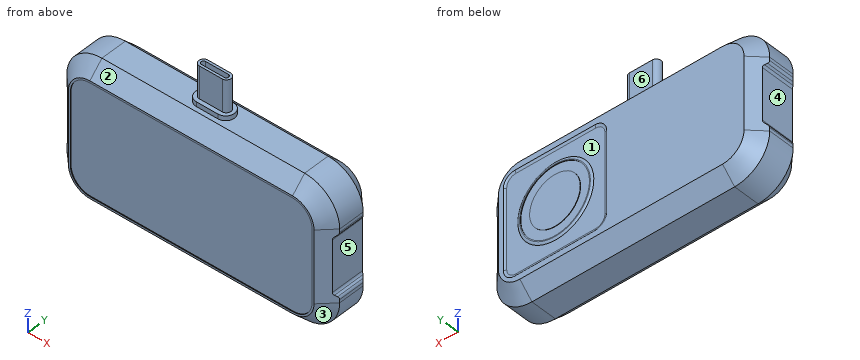
```python
from build123d import *

# Parameters (mm, degrees)
SKETCH1_W               = 70
SKETCH1_H               = 36.5
BOSS_EXTRUDE1_DEPTH     = 6.9
BOSS_EXTRUDE2_DEPTH     = 1.2
BOSS_EXTRUDE3_DEPTH     = 8.25
FILLET1_R               = 9
SKETCH4_R               = 9.75
CUT_EXTRUDE1_DEPTH      = 0.25
SKETCH5_R               = 8.85
SKETCH5_R_2             = 6.5
CUT_EXTRUDE2_DEPTH      = 0.1
CHAMFER1_SIZE           = 3.5
CUT_EXTRUDE3_DEPTH      = 0.2
CUT_EXTRUDE4_DEPTH      = 46.16525213
CUT_EXTRUDE4_DEPTH_BACK = 46.16525213
FILLET2_R               = 1
FILLET3_R               = 1


with BuildPart() as part:
    # Sketch1 → Boss-Extrude1 (new, symmetric)
    with BuildSketch(Plane(origin=(0, 0, 0), x_dir=(1, 0, 0), z_dir=(0, 1, 0))):
        Rectangle(SKETCH1_W, SKETCH1_H)
    extrude(amount=BOSS_EXTRUDE1_DEPTH, both=True)

    # Sketch2 → Boss-Extrude2 (add)
    with BuildSketch(Plane.XY.offset(18.25)):
        with BuildLine():
            Line((2.75, -2.25), (-2.75, -2.25))
            ThreePointArc((-2.75, -2.25), (-5, 0), (-2.75, 2.25))
            Line((-2.75, 2.25), (2.75, 2.25))
            ThreePointArc((2.75, 2.25), (5, 0), (2.75, -2.25))
        make_face()
    extrude(amount=BOSS_EXTRUDE2_DEPTH)

    # Sketch3 → Boss-Extrude3 (add)
    with BuildSketch(Plane.XY.offset(19.45)):
        with BuildLine():
            Line((2.925, -1.2), (-2.925, -1.2))
            ThreePointArc((-2.925, -1.2), (-4.125, 0), (-2.925, 1.2))
            Line((-2.925, 1.2), (2.925, 1.2))
            ThreePointArc((2.925, 1.2), (4.125, 0), (2.925, -1.2))
        make_face()
        with BuildLine():
            Line((2.925, -0.6), (-2.925, -0.6))
            ThreePointArc((-2.925, -0.6), (-3.525, 0), (-2.925, 0.6))
            Line((-2.925, 0.6), (2.925, 0.6))
            ThreePointArc((2.925, 0.6), (3.525, 0), (2.925, -0.6))
        make_face(mode=Mode.SUBTRACT)
    extrude(amount=BOSS_EXTRUDE3_DEPTH)

    # Fillet1
    fillet1_edges = [part.edges().sort_by_distance(p)[0] for p in [
        (35, 0, 18.25),
        (-35, 0, 18.25),
        (-35, 0, -18.25),
        (35, 0, -18.25),
    ]]
    fillet(fillet1_edges, radius=FILLET1_R)

    # Sketch4 → Cut-Extrude1 (cut)
    with BuildSketch(Plane(origin=(0, 6.9, 0), x_dir=(1, 0, 0), z_dir=(0, 1, 0))):
        with BuildLine():
            Line((27.25, 13.25), (6.75, 13.25))
            ThreePointArc((6.75, 13.25), (4.628679656, 12.371320344), (3.75, 10.25))
            Line((3.75, 10.25), (3.75, -10.25))
            ThreePointArc((3.75, -10.25), (4.628679656, -12.371320344), (6.75, -13.25))
            Line((6.75, -13.25), (27.25, -13.25))
            ThreePointArc((27.25, -13.25), (29.371320344, -12.371320344), (30.25, -10.25))
            Line((30.25, -10.25), (30.25, 10.25))
            ThreePointArc((30.25, 10.25), (29.371320344, 12.371320344), (27.25, 13.25))
        make_face()
        with Locations(Location((17, 0, 0), (0, 0, 270))):
            Circle(SKETCH4_R, mode=Mode.SUBTRACT)
    extrude(amount=-CUT_EXTRUDE1_DEPTH, mode=Mode.SUBTRACT)

    # Sketch5 → Cut-Extrude2 (cut)
    with BuildSketch(Plane(origin=(0, 6.9, 0), x_dir=(1, 0, 0), z_dir=(0, 1, 0))):
        with Locations(Location((17, 0, 0), (0, 0, 270))):
            Circle(SKETCH5_R)
        with Locations(Location((17, 0, 0), (0, 0, 270))):
            Circle(SKETCH5_R_2, mode=Mode.SUBTRACT)
    extrude(amount=-CUT_EXTRUDE2_DEPTH, mode=Mode.SUBTRACT)

    # Chamfer1
    chamfer1_edges = [part.edges().sort_by_distance(p)[0] for p in [
        (0, -6.9, -18.25),
        (0, 6.9, -18.25),
        (35, -6.9, 0),
        (0, -6.9, 18.25),
        (-35, -6.9, 0),
        (-32.363961031, -6.9, 15.613961031),
        (-32.363961031, -6.9, -15.613961031),
        (32.363961031, -6.9, 15.613961031),
        (32.363961031, -6.9, -15.613961031),
        (35, 6.9, 0),
        (-35, 6.9, 0),
        (0, 6.9, 18.25),
        (-32.363961031, 6.9, 15.613961031),
        (-32.363961031, 6.9, -15.613961031),
        (32.363961031, 6.9, 15.613961031),
        (32.363961031, 6.9, -15.613961031),
    ]]
    chamfer(chamfer1_edges, length=CHAMFER1_SIZE)

    # Sketch6 → Cut-Extrude3 (cut)
    with BuildSketch(Plane.XZ.offset(6.9)):
        with BuildLine():
            Line((-26, -14.25), (26, -14.25))
            ThreePointArc((26, -14.25), (29.535533906, -12.785533906), (31, -9.25))
            Line((31, -9.25), (31, 9.25))
            ThreePointArc((31, 9.25), (29.535533906, 12.785533906), (26, 14.25))
            Line((26, 14.25), (-26, 14.25))
            ThreePointArc((-26, 14.25), (-29.535533906, 12.785533906), (-31, 9.25))
            Line((-31, 9.25), (-31, -9.25))
            ThreePointArc((-31, -9.25), (-29.535533906, -12.785533906), (-26, -14.25))
        make_face()
    extrude(amount=-CUT_EXTRUDE3_DEPTH, mode=Mode.SUBTRACT)

    # Sketch7 → Cut-Extrude4 (cut, two sides: drawn at the far end of the back side and taken through both)
    with BuildSketch(Plane(origin=(0, 0, 0), x_dir=(1, 0, 0), z_dir=(0, 1, 0)).offset(-CUT_EXTRUDE4_DEPTH_BACK)):
        Polygon((-34, -7), (-34, 7), (-35, 8), (-35, -8), align=None)
        Polygon((34, 7), (35, 8), (35, -8), (34, -7), align=None)
    extrude(amount=CUT_EXTRUDE4_DEPTH + CUT_EXTRUDE4_DEPTH_BACK, mode=Mode.SUBTRACT)

    # Fillet2
    fillet2_edges = [part.edges().sort_by_distance(p)[0] for p in [
        (34, 0, 7),
        (34, 0, -7),
        (35, 0, -8),
        (35, 0, 8),
        (-35, 0, -8),
        (-34, 0, -7),
        (-34, 0, 7),
        (-35, 0, 8),
    ]]
    fillet(fillet2_edges, radius=FILLET2_R)

    # Fillet3
    # the kernel refuses this fillet: 1 mm, written as the material it adds along each edge
    with BuildSketch(Plane(origin=(27.25, 6.65, -10.25), x_dir=(1, 0, 0), z_dir=(0, 0, 1))) as fillet3_piece_1:
        with BuildLine():
            CenterArc((2.338562172, 1), FILLET3_R, 270, 41.409622109)
            Line((2.338562172, 0), (2.338562172, -0.02))
            Line((2.338562172, -0.02), (3, -0.02))
            Line((3, -0.02), (3.02, 0))
            ThreePointArc((3.02, 0), (3.02, 0.125), (3.013228757, 0.235))
            Line((3.013228757, 0.235), (3, 0.25))
        make_face()
    revolve(axis=Axis((27.25, 6.65, -10.25), (0, 1, 0)), revolution_arc=90)
    with BuildSketch(Plane(origin=(30.25, 6.65, 10.25), x_dir=(0, 1, 0), z_dir=(0, 0, -1)), Plane(origin=(6.75, 6.65, 13.25), x_dir=(0, 1, 0), z_dir=(1, 0, 0)), Plane(origin=(3.75, 6.65, -10.25), x_dir=(0, 1, 0), z_dir=(0, 0, 1)), Plane(origin=(27.25, 6.65, -13.25), x_dir=(0, 1, 0), z_dir=(-1, 0, 0))) as fillet3_piece_2:
        with BuildLine():
            CenterArc((1, -0.661437828), FILLET3_R, 138.590377891, 41.409622109)
            Line((0, -0.661437828), (-0.02, -0.661437828))
            Line((-0.02, -0.661437828), (-0.02, 0))
            Line((-0.02, 0), (0, 0.02))
            ThreePointArc((0, 0.02), (0.125, 0.02), (0.235, 0.013228757))
            Line((0.235, 0.013228757), (0.25, 0))
        make_face()
    extrude(amount=20.5)
    with BuildSketch(Plane(origin=(27.25, 6.65, 10.25), x_dir=(0, 0, 1), z_dir=(-1, 0, 0))) as fillet3_piece_3:
        with BuildLine():
            CenterArc((2.338562172, 1), FILLET3_R, 270, 41.409622109)
            Line((2.338562172, 0), (2.338562172, -0.02))
            Line((2.338562172, -0.02), (3, -0.02))
            Line((3, -0.02), (3.02, 0))
            ThreePointArc((3.02, 0), (3.02, 0.125), (3.013228757, 0.235))
            Line((3.013228757, 0.235), (3, 0.25))
        make_face()
    revolve(axis=Axis((27.25, 6.65, 10.25), (0, 1, 0)), revolution_arc=90)
    with BuildSketch(Plane(origin=(6.75, 6.65, 10.25), x_dir=(-1, 0, 0), z_dir=(0, 0, -1))) as fillet3_piece_4:
        with BuildLine():
            CenterArc((2.338562172, 1), FILLET3_R, 270, 41.409622109)
            Line((2.338562172, 0), (2.338562172, -0.02))
            Line((2.338562172, -0.02), (3, -0.02))
            Line((3, -0.02), (3.02, 0))
            ThreePointArc((3.02, 0), (3.02, 0.125), (3.013228757, 0.235))
            Line((3.013228757, 0.235), (3, 0.25))
        make_face()
    revolve(axis=Axis((6.75, 6.65, 10.25), (0, 1, 0)), revolution_arc=90)
    with BuildSketch(Plane(origin=(6.75, 6.65, -10.25), x_dir=(0, 0, -1), z_dir=(1, 0, 0))) as fillet3_piece_5:
        with BuildLine():
            CenterArc((2.338562172, 1), FILLET3_R, 270, 41.409622109)
            Line((2.338562172, 0), (2.338562172, -0.02))
            Line((2.338562172, -0.02), (3, -0.02))
            Line((3, -0.02), (3.02, 0))
            ThreePointArc((3.02, 0), (3.02, 0.125), (3.013228757, 0.235))
            Line((3.013228757, 0.235), (3, 0.25))
        make_face()
    revolve(axis=Axis((6.75, 6.65, -10.25), (0, 1, 0)), revolution_arc=90)
    # the kernel refuses this fillet: 1 mm, written as the material it takes off along each edge
    with BuildSketch(Plane(origin=(17, 6.9, 0), x_dir=(0, 0, 1), z_dir=(-1, 0, 0))) as fillet3_2_piece_1:
        with BuildLine():
            CenterArc((9.088562172, -1), FILLET3_R, 48.590377891, 41.409622109)
            Line((9.088562172, 0), (9.088562172, 0.02))
            Line((9.088562172, 0.02), (9.75, 0.02))
            Line((9.75, 0.02), (9.77, 0))
            ThreePointArc((9.77, 0), (9.77, -0.125), (9.763228757, -0.235))
            Line((9.763228757, -0.235), (9.75, -0.25))
        make_face()
    revolve(axis=Axis((17, 6.9, 0), (0, 1, 0)), mode=Mode.SUBTRACT)


solid = part.part
```
Here's how the part is built. I have some questions about the finished solid (model axes, mm). Face numbers are marked on the shaded views. A direction names the side the tool comes from. Give positions to 0.01 mm unless a question says otherwise; leave off trailing zeros. Write each loop counter-clockwise with the first axis right and the second up, starting at its lowest first coordinate (ties: lowest second). Pieces come first, ordered by that corner, then holes. Notation, with made-up numbers: (10, 86) -> (36, 86) arc R19 cw to (36, 103) -> close; hole circle Ø3 at (-5, -36.75). An arc over 180 degrees is marked (long way). Write each question's results on one line, items separated by ' | '.
Item 1: Suppose I cut it at B-B on x = 17. Write out the boundary of the cut face in (y, z), plus the area to 3 significant figures.
Output:
outline: (-6.9, -14.75) -> (-3.4, -18.25) -> (3.4, -18.25) -> (6.9, -14.75) -> (6.9, -13.25) arc R1 cw to (6.65, -12.59) -> (6.65, -9.75) arc R1 ccw to (6.9, -9.09) -> (6.9, -8.85) -> (6.8, -8.85) -> (6.8, -6.5) -> (6.9, -6.5) -> (6.9, 6.5) -> (6.8, 6.5) -> (6.8, 8.85) -> (6.9, 8.85) -> (6.9, 9.09) arc R1 ccw to (6.65, 9.75) -> (6.65, 12.59) arc R1 cw to (6.9, 13.25) -> (6.9, 14.75) -> (3.4, 18.25) -> (-3.4, 18.25) -> (-6.9, 14.75) -> (-6.9, 14.25) -> (-6.7, 14.25) -> (-6.7, -14.25) -> (-6.9, -14.25) -> close | area: 471 mm^2
Item 2: Suppose I cut it at A-A on y = 5.25. Write out the boundary of the cut face in (x, z).
Output:
outline: (-33.15, -9.25) arc R7.15 ccw to (-26, -16.4) -> (26, -16.4) arc R7.15 ccw to (33.15, -9.25) -> (33.15, 9.25) arc R7.15 ccw to (26, 16.4) -> (-26, 16.4) arc R7.15 ccw to (-33.15, 9.25) -> close
Item 3: On a 3-axis mill with a long thin cutter (end or side, diameter ignored), from which of +Z, -Z, +X, -X, +Y, -Y can I reach the whole of each face in a straight line? I mean the marked faces 4, 5 and 6. Say none if no direction works.
Output:
face 4: -X, +Y, -Y | face 5: +X, +Y, -Y | face 6: +Z, +X, -X, +Y
Item 4: For pin 1 Ø6 at (y, z) = (2, 19.5) entering from +X; pin 2 Ø6.5 at (x, z) = (1, 24) entering from -Y; pin 3 Ø1 at (x, z) = (1.5, 18.5) entering from -Y, each with a flat end and sliding along its axis, tell me the tip position at first contact or that it passes through.
Output:
pin 1: stops at x = 31.33 | pin 2: stops at y = -1.2 | pin 3: stops at y = -3.65
Item 5: If I drill on L1, parallel to X at y = 1.25, z = 4.5; L2, parallel to Y at x = -18, z = 4.5; L3, parallel to Z at x = 15, y = -1.5, over which ranges is the centre line in solid material (lowest first)?
Output:
L1: x = -34 to 34 | L2: y = -6.7 to 6.9 | L3: z = -18.25 to 18.25
Item 6: Suppose I cut it at C-C on x = -12.5. Write out the boundary of the cut face in (y, z), plus the area to 4 significant figures.
Output:
outline: (-6.9, -14.75) -> (-3.4, -18.25) -> (3.4, -18.25) -> (6.9, -14.75) -> (6.9, 14.75) -> (3.4, 18.25) -> (-3.4, 18.25) -> (-6.9, 14.75) -> (-6.9, 14.25) -> (-6.7, 14.25) -> (-6.7, -14.25) -> (-6.9, -14.25) -> close | area: 473.5 mm^2
Item 7: We'd pull the mould along Z, two halves only. Please class the marked faces 1, 2 and 3: pulls with the +Z half, pulls with the -Z half, needs draft (parallel to the pull), parting line crosses it, or undercut.
Output:
face 1: undercut | face 2: pulls with the +Z half | face 3: pulls with the -Z half
Item 8: Suppose I cut it at D-D on x = -1. Write out the boundary of the cut face in (y, z).
Output:
outline: (-6.9, -14.75) -> (-3.4, -18.25) -> (3.4, -18.25) -> (6.9, -14.75) -> (6.9, 14.75) -> (3.4, 18.25) -> (2.25, 18.25) -> (2.25, 19.45) -> (1.2, 19.45) -> (1.2, 27.7) -> (0.6, 27.7) -> (0.6, 19.45) -> (-0.6, 19.45) -> (-0.6, 27.7) -> (-1.2, 27.7) -> (-1.2, 19.45) -> (-2.25, 19.45) -> (-2.25, 18.25) -> (-3.4, 18.25) -> (-6.9, 14.75) -> (-6.9, 14.25) -> (-6.7, 14.25) -> (-6.7, -14.25) -> (-6.9, -14.25) -> close
